from build123d import *

# Parameters (mm, degrees)
SKETCH1_W           = 12.7
SKETCH1_H           = 12.7
BOSS_EXTRUDE1_DEPTH = 177.8
SKETCH2_R           = 6.35
BOSS_EXTRUDE2_DEPTH = 25.4
SKETCH3_W           = 12.7
SKETCH3_H           = 158.75
BOSS_EXTRUDE3_DEPTH = 28.652
BOSS_EXTRUDE4_START = 19.05
SKETCH4_W           = 12.7
SKETCH4_H           = 19.05
BOSS_EXTRUDE4_DEPTH = 9.602
CUT_EXTRUDE1_START  = -4
SKETCH5_R           = 1.274448637
CUT_EXTRUDE1_DEPTH  = 4
CUT_EXTRUDE2_START  = -6.35
SKETCH5_2_R         = 1.274448637
CUT_EXTRUDE2_DEPTH  = 6.35
SKETCH8_W           = 9.448
SKETCH8_H           = 31.75
SKETCH8_W_2         = 50.8
BOSS_EXTRUDE5_DEPTH = 12.7
SKETCH8_3_W         = 9.448
SKETCH8_3_H         = 31.75
SKETCH8_3_W_2       = 50.8
BOSS_EXTRUDE6_DEPTH = 15.24
SKETCH9_W           = 41.402
SKETCH9_H           = 20.066
CUT_EXTRUDE3_DEPTH  = 21.082
SKETCH7_W           = 12.7
SKETCH7_H           = 16.764
BOSS_EXTRUDE7_DEPTH = 12.7
BOSS_EXTRUDE8_START = -38.1
BOSS_EXTRUDE8_DEPTH = 12.7
SKETCH10_W          = 3.962
SKETCH10_H          = 19.562
SKETCH10_W_2        = 3.2
SKETCH10_H_2        = 18.8
SKETCH10_W_3        = 2.372565257
SKETCH10_H_3        = 2.262
CUT_EXTRUDE4_DEPTH  = 207.185481547


with BuildPart() as part:
    # Sketch1 → Boss-Extrude1 (new body)
    with BuildSketch(Plane(origin=(0, 0, 0), x_dir=(1, 0, 0), z_dir=(0, 1, 0))):
        Rectangle(SKETCH1_W, SKETCH1_H)
    extrude(amount=-BOSS_EXTRUDE1_DEPTH)

    # Sketch2 → Boss-Extrude2 (add, symmetric)
    with BuildSketch(Plane(origin=(0, 0, 0), x_dir=(0, 0, -1), z_dir=(1, 0, 0))):
        with Locations((0, -6.35)):
            Circle(SKETCH2_R)
    extrude(amount=BOSS_EXTRUDE2_DEPTH, both=True)

    # Sketch3 → Boss-Extrude3 (add)
    with BuildSketch(Plane.ZY.offset(6.35)):
        with Locations((0, -98.425)):
            Rectangle(SKETCH3_W, SKETCH3_H)
    extrude(amount=BOSS_EXTRUDE3_DEPTH)

    # Sketch4 → Boss-Extrude4 (add)
    with BuildSketch(Plane.ZY.offset(6.35).offset(BOSS_EXTRUDE4_START)):
        with Locations((0, -9.525)):
            Rectangle(SKETCH4_W, SKETCH4_H)
    extrude(amount=BOSS_EXTRUDE4_DEPTH)

    # Sketch5 → Cut-Extrude1 (cut)
    with BuildSketch(Plane.ZY.offset(35.002).offset(CUT_EXTRUDE1_START)):
        with BuildLine():
            Line((-3.833, -30.756), (-3.833, -16.606))
            ThreePointArc((-3.833, -16.606), (-4.34616702, -13.44372234), (-5.833, -10.606))
            ThreePointArc((-5.833, -10.606), (-6.104434225, -10.218346078), (-6.35, -9.81380986))
            Line((-6.35, -9.81380986), (-6.35, 0))
            Line((-6.35, 0), (-3.697009279, 0))
            Line((-3.697009279, 0), (3.631009279, 0))
            Line((3.631009279, 0), (6.35, 0))
            Line((6.35, 0), (6.35, -9.693995201))
            ThreePointArc((6.35, -9.693995201), (6.075544052, -10.160893028), (5.767, -10.606))
            ThreePointArc((5.767, -10.606), (4.280167019, -13.44372234), (3.767, -16.606))
            Line((3.767, -16.606), (3.767, -30.756))
            ThreePointArc((3.767, -30.756), (-0.033, -34.556), (-3.833, -30.756))
        make_face()
        with Locations(Location((-0.033, -26.756, 0), (0, 0, 270))):
            Circle(SKETCH5_R, mode=Mode.SUBTRACT)
        with Locations(Location((-0.033, -30.756, 0), (0, 0, 270))):
            Circle(SKETCH5_R, mode=Mode.SUBTRACT)
    extrude(amount=CUT_EXTRUDE1_DEPTH, mode=Mode.SUBTRACT)

    # Sketch5<2> → Cut-Extrude2 (cut)
    with BuildSketch(Plane.ZY.offset(35.002).offset(CUT_EXTRUDE2_START)):
        with Locations(Location((-0.033, -26.756, 0), (0, 0, 270))):
            Circle(SKETCH5_2_R)
        with Locations(Location((-0.033, -30.756, 0), (0, 0, 270))):
            Circle(SKETCH5_2_R)
    extrude(amount=CUT_EXTRUDE2_DEPTH, mode=Mode.SUBTRACT)

    # Sketch8 → Boss-Extrude5 (add)
    with BuildSketch(Plane.XY.offset(6.35)):
        with Locations((-39.726, -161.925)):
            Rectangle(SKETCH8_W, SKETCH8_H)
        with Locations((-69.85, -161.925)):
            Rectangle(SKETCH8_W_2, SKETCH8_H)
    extrude(amount=-BOSS_EXTRUDE5_DEPTH)

    # Sketch8<3> → Boss-Extrude6 (add)
    with BuildSketch(Plane.XY.offset(6.35)):
        with Locations((-39.726, -161.925)):
            Rectangle(SKETCH8_3_W, SKETCH8_3_H)
        with Locations((-69.85, -161.925)):
            Rectangle(SKETCH8_3_W_2, SKETCH8_3_H)
    extrude(amount=BOSS_EXTRUDE6_DEPTH)

    # Sketch9 → Cut-Extrude3 (cut)
    with BuildSketch(Plane(origin=(0, 0, -6.35), x_dir=(-1, 0, 0), z_dir=(0, 0, -1))):
        with Locations((65.151, -161.925)):
            Rectangle(SKETCH9_W, SKETCH9_H)
    extrude(amount=-CUT_EXTRUDE3_DEPTH, mode=Mode.SUBTRACT)

    # Sketch7 → Boss-Extrude7 (add)
    with BuildSketch(Plane(origin=(6.35, 0, 0), x_dir=(0, 0, -1), z_dir=(1, 0, 0))):
        with BuildLine():
            Line((6.35, -153.67), (6.35, -170.434))
            Line((6.35, -170.434), (15.24, -170.434))
            ThreePointArc((15.24, -170.434), (18.221863859, -169.885671676), (20.813596386, -168.312427088))
            ThreePointArc((20.813596386, -168.312427088), (20.896848593, -166.878), (19.462421505, -166.794747794))
            ThreePointArc((19.462421505, -166.794747794), (8.89, -162.052), (19.462421505, -157.309252206))
            Line((19.462421505, -157.309252206), (20.813596386, -155.791572912))
            ThreePointArc((20.813596386, -155.791572912), (18.221863859, -154.218328324), (15.24, -153.67))
            Line((15.24, -153.67), (6.35, -153.67))
        make_face()
        with Locations((0, -162.052)):
            Rectangle(SKETCH7_W, SKETCH7_H)
        with BuildLine():
            ThreePointArc((19.462421505, -157.309252206), (20.896848593, -157.226), (20.813596386, -155.791572912))
            Line((20.813596386, -155.791572912), (19.462421505, -157.309252206))
        make_face()
    extrude(amount=BOSS_EXTRUDE7_DEPTH)

    # Sketch7<4> → Boss-Extrude8 (add)
    with BuildSketch(Plane(origin=(6.35, 0, 0), x_dir=(0, 0, -1), z_dir=(1, 0, 0)).offset(BOSS_EXTRUDE8_START)):
        with BuildLine():
            Line((6.35, -153.67), (6.35, -170.434))
            Line((6.35, -170.434), (15.24, -170.434))
            ThreePointArc((15.24, -170.434), (18.221863859, -169.885671676), (20.813596386, -168.312427088))
            ThreePointArc((20.813596386, -168.312427088), (20.896848593, -166.878), (19.462421505, -166.794747794))
            ThreePointArc((19.462421505, -166.794747794), (8.89, -162.052), (19.462421505, -157.309252206))
            ThreePointArc((19.462421505, -157.309252206), (20.896848593, -157.226), (20.813596386, -155.791572912))
            ThreePointArc((20.813596386, -155.791572912), (18.221863859, -154.218328324), (15.24, -153.67))
            Line((15.24, -153.67), (6.35, -153.67))
        make_face()
    extrude(amount=BOSS_EXTRUDE8_DEPTH)

    # Sketch10 → Cut-Extrude4 (cut, through all)
    # profile 1 of 2: a face of its own
    with BuildSketch(Plane.XY.offset(21.59)):
        with Locations((-56.752, -161.958)):
            Rectangle(SKETCH10_W, SKETCH10_H)
        with Locations((-56.752, -161.958)):
            Rectangle(SKETCH10_W_2, SKETCH10_H_2, mode=Mode.SUBTRACT)
    # profile 2 of 2: a face of its own
    with BuildSketch(Plane.XY.offset(21.59)):
        with Locations((-53.965717372, -161.958)):
            Rectangle(SKETCH10_W_3, SKETCH10_H_3)
    extrude(amount=-CUT_EXTRUDE4_DEPTH, mode=Mode.SUBTRACT)


with BuildPart() as cut_extrude4_kept_piece:
    # of the separate pieces the step leaves, the one the design keeps (cut_extrude4_pieces_kept)
    add(part.part.solids().sort_by_distance((-6.35, 0, 6.35))[0])


solid = cut_extrude4_kept_piece.part
Input: part model. Units: mm. Frame: model coordinates. A direction names the side the tool comes from. Coordinates: 2 decimals unless noted, no trailing zeros. Loops run counter-clockwise (first coordinate to the right, second up) from the corner with the lowest first, then second, coordinate; pieces in that order, holes last. Notation, with made-up numbers: (20, 0.25) -> (74, 0.25) arc R14 cw to (74, 17.25) -> close; hole circle Ø7 at (43, -25.75). An arc over 180 degrees is marked (long way). Write each question's results on one line, items separated by ' | '. Start each with the question number.
Q1. Ray query, line 1 (Y direction, x = -23, z = -15.24); line 2 (X direction, y = -156, z = -7); line 3 (Y direction, x = -59.5, z = 13.5). Return the intervals inside material, ascending. Write a range as from..to.
Q2. Section B-B, the plane x = -83. Return the cut outline in (y, z), plus the area to 3 significant figures.
Q3. Section A-A, the plane z = 18. Return the cut outline in (x, y), plus the area to 3 significant figures.
Q4. Section D-D, the plane y = -118. Return the cut outline in (x, z), plus the area to 3 significant figures.
Q5. Pin query (flat end, axial travel): pin 1 (7 mm diameter, centred on y = -3.5, z = 4, fed in from -X); pin 2 (0.8 mm diameter, centred on y = -31, z = 0, fed in from -X); pin 3 (16.5 mm diameter, centred on y = -162.5, z = -16, fed in from +X); pin 4 (11.5 mm diameter, centred on y = -162.052, z = -15.24, fed in from +X). Return the tip coordinate at first contact, or that it passes through.
Q6. Pull-direction query (Z, two-part tool) for faces 4 (the cylindrical face through (16.01, -10.21, 5.04)), 5 (the cylindrical face through (-25.489, -162.256, -8.893)), 6 (the flat face through (-35.002, -162, 14)); classes: released by +Z, released by -Z, zero draft, split by the parting line, or undercut.
Q7. Reachability of faces 1 (the cylindrical face through (-32.97, -13.49, -4.33)), 2 (the flat face through (-25, -170.434, -11)), 3 (the flat face through (19.05, -162, -4)) from +Z, -Z, +X, -X, +Y, -Y: full face, straight path, thin tool, end or side. Return the list, or none.
Q8. Section C-C, the plane x = 16. Return the cut outline in (y, z).
Found:
1) line 1: -170.43..-168.4, -155.7..-153.67 | line 2: -31.75..-19.05, 6.35..19.05 | line 3: -177.8..-171.96, -151.89..-146.05
2) outline: (-177.8, -6.35) -> (-171.96, -6.35) -> (-171.96, 14.73) -> (-151.89, 14.73) -> (-151.89, -6.35) -> (-146.05, -6.35) -> (-146.05, 21.59) -> (-177.8, 21.59) -> close | area: 464 mm2
3) outline: (-95.25, -177.8) -> (-35, -177.8) -> (-35, -146.05) -> (-95.25, -146.05) -> close; hole (-58.73, -171.74) -> (-54.77, -171.74) -> (-54.77, -163.09) -> (-52.78, -163.09) -> (-52.78, -160.83) -> (-54.77, -160.83) -> (-54.77, -152.18) -> (-58.73, -152.18) -> close | area: 1,830 mm2
4) outline: (-35, -6.35) -> (6.35, -6.35) -> (6.35, 6.35) -> (-35, 6.35) -> close | area: 525 mm2
5) pin 1: x = -31 | pin 2: x = -28.65 | pin 3: x = 19.05 | pin 4: through
6) face 4: split by the parting line | face 5: undercut | face 6: zero draft
7) face 1: -X, +Y | face 2: -Z, +X, -X, -Y | face 3: +Z, -Z, +X, -Y
8) outline: (-170.43, -15.24) arc R8.38 ccw to (-168.31, -20.81) arc R1.02 ccw to (-166.79, -19.46) arc R6.35 cw (long way) to (-157.31, -19.46) arc R1.02 ccw to (-155.79, -20.81) arc R8.38 ccw to (-153.67, -15.24) -> (-153.67, 6.35) -> (-170.43, 6.35) -> close; circle Ø12.7 at (-6.35, 0)
